CAD build for the part. Positions are in the model's coordinates, mm. Round coordinates to 2 decimals unless told otherwise and drop trailing zeros. Answer as CSV lines item,"result". Start each with the question number.
from build123d import *

# Parameters (mm, degrees)
SKETCH_R  = 2.1
PAD_DEPTH = 800


with BuildPart() as part:
    # Sketch → Pad (new body)
    with BuildSketch(Plane.XY):
        with BuildLine():
            Line((-10, 4.58), (-10, 9.5))
            ThreePointArc((-9.5, 10), (-9.853553, 9.853553), (-10, 9.5))
            Line((-9.5, 10), (-4.58, 10))
            Line((-4.58, 10), (-3.125, 8.545))
            Line((-3.125, 8.545), (-3.125, 8.2))
            Line((-5.5, 8.2), (-3.125, 8.2))
            Line((-5.5, 8.2), (-5.5, 6.56066))
            Line((-5.5, 6.56066), (-2.83934, 3.9))
            Line((-0.125, 3.9), (-2.83934, 3.9))
            ThreePointArc((-0.125, 3.9), (0, 3.775), (0.125, 3.9))
            Line((0.125, 3.9), (2.83934, 3.9))
            Line((2.83934, 3.9), (5.5, 6.56066))
            Line((5.5, 6.56066), (5.5, 8.2))
            Line((5.5, 8.2), (3.125, 8.2))
            Line((3.125, 8.2), (3.125, 8.545))
            Line((3.125, 8.545), (4.58, 10))
            Line((4.58, 10), (15.42, 10))
            Line((15.42, 10), (16.875, 8.545))
            Line((16.875, 8.545), (16.875, 8.2))
            Line((16.875, 8.2), (14.5, 8.2))
            Line((14.5, 8.2), (14.5, 6.56066))
            Line((14.5, 6.56066), (17.16066, 3.9))
            Line((17.16066, 3.9), (19.875, 3.9))
            ThreePointArc((19.875, 3.9), (20, 3.775), (20.125, 3.9))
            Line((20.125, 3.9), (22.83934, 3.9))
            Line((22.83934, 3.9), (25.5, 6.56066))
            Line((25.5, 6.56066), (25.5, 8.2))
            Line((25.5, 8.2), (23.125, 8.2))
            Line((23.125, 8.2), (23.125, 8.545))
            Line((23.125, 8.545), (24.58, 10))
            Line((24.58, 10), (29.5, 10))
            ThreePointArc((30, 9.5), (29.853554, 9.853554), (29.5, 10))
            Line((30, 9.5), (30, 4.58))
            Line((30, 4.58), (28.545, 3.125))
            Line((28.545, 3.125), (28.2, 3.125))
            Line((28.2, 3.125), (28.2, 5.5))
            Line((28.2, 5.5), (26.560661, 5.5))
            Line((26.560661, 5.5), (23.9, 2.83934))
            Line((23.9, 2.83934), (23.9, 0.125))
            ThreePointArc((23.9, 0.125), (23.775, 2e-06), (23.899997, -0.125))
            Line((23.899997, -2.83934), (23.899997, -0.125))
            Line((26.560658, -5.5), (23.899997, -2.83934))
            Line((28.199997, -5.5), (26.560658, -5.5))
            Line((28.199997, -3.125), (28.199997, -5.5))
            Line((28.544997, -3.125), (28.199997, -3.125))
            Line((29.999997, -4.58), (28.544997, -3.125))
            Line((29.999997, -9.5), (29.999997, -4.58))
            ThreePointArc((29.5, -10), (29.853552, -9.853552), (29.999997, -9.5))
            Line((24.58, -10), (29.5, -10))
            Line((23.125, -8.545), (24.58, -10))
            Line((23.125, -8.2), (23.125, -8.545))
            Line((25.5, -8.2), (23.125, -8.2))
            Line((25.5, -6.56066), (25.5, -8.2))
            Line((22.83934, -3.9), (25.5, -6.56066))
            Line((20.125, -3.9), (22.83934, -3.9))
            ThreePointArc((20.125, -3.9), (20, -3.775), (19.875, -3.9))
            Line((17.16066, -3.9), (19.875, -3.9))
            Line((14.5, -6.56066), (17.16066, -3.9))
            Line((14.5, -8.2), (14.5, -6.56066))
            Line((16.875, -8.2), (14.5, -8.2))
            Line((16.875, -8.545), (16.875, -8.2))
            Line((15.42, -10), (16.875, -8.545))
            Line((4.58, -10), (15.42, -10))
            Line((4.58, -10), (3.125, -8.545))
            Line((3.125, -8.545), (3.125, -8.2))
            Line((3.125, -8.2), (5.5, -8.2))
            Line((5.5, -8.2), (5.5, -6.56066))
            Line((2.83934, -3.9), (5.5, -6.56066))
            Line((0.125, -3.9), (2.83934, -3.9))
            ThreePointArc((0.125, -3.9), (0, -3.775), (-0.125, -3.9))
            Line((-0.125, -3.9), (-2.83934, -3.9))
            Line((-2.83934, -3.9), (-5.5, -6.56066))
            Line((-5.5, -6.56066), (-5.5, -8.2))
            Line((-5.5, -8.2), (-3.125, -8.2))
            Line((-3.125, -8.545), (-3.125, -8.2))
            Line((-4.58, -10), (-3.125, -8.545))
            Line((-9.5, -10), (-4.58, -10))
            ThreePointArc((-10, -9.5), (-9.853553, -9.853553), (-9.5, -10))
            Line((-10, -4.58), (-10, -9.5))
            Line((-8.545, -3.125), (-10, -4.58))
            Line((-8.2, -3.125), (-8.545, -3.125))
            Line((-8.2, -5.5), (-8.2, -3.125))
            Line((-6.56066, -5.5), (-8.2, -5.5))
            Line((-3.9, -2.83934), (-6.56066, -5.5))
            Line((-3.9, -0.125), (-3.9, -2.83934))
            ThreePointArc((-3.9, -0.125), (-3.775, 0), (-3.9, 0.125))
            Line((-3.9, 2.83934), (-3.9, 0.125))
            Line((-6.56066, 5.5), (-3.9, 2.83934))
            Line((-8.2, 5.5), (-6.56066, 5.5))
            Line((-8.2, 5.5), (-8.2, 3.125))
            Line((-8.545, 3.125), (-8.2, 3.125))
            Line((-10, 4.58), (-8.545, 3.125))
        make_face()
        Circle(SKETCH_R, mode=Mode.SUBTRACT)
        with Locations((20, 0)):
            Circle(SKETCH_R, mode=Mode.SUBTRACT)
        with BuildLine():
            Line((7, 5.93934), (3.9, 2.83934))
            Line((3.9, 2.83934), (3.9, 0.125))
            ThreePointArc((3.9, 0.125), (3.775, 0), (3.9, -0.125))
            Line((3.9, -0.125), (3.9, -2.83934))
            Line((3.9, -2.83934), (7, -5.93934))
            Line((7, -5.93934), (7, -8.2))
            Line((7, -8.2), (13, -8.2))
            Line((13, -8.2), (13, -5.93934))
            Line((13, -5.93934), (16.1, -2.83934))
            Line((16.1, -2.83934), (16.1, -0.125))
            ThreePointArc((16.1, -0.125), (16.224999, 0), (16.1, 0.125))
            Line((16.1, 2.83934), (16.1, 0.125))
            Line((13, 5.93934), (16.1, 2.83934))
            Line((13, 8.2), (13, 5.93934))
            Line((7, 8.2), (13, 8.2))
            Line((7, 5.93934), (7, 8.2))
        make_face(mode=Mode.SUBTRACT)
    extrude(amount=PAD_DEPTH)


solid = part.part
Item 1: Probe line 1 (X direction, y = 6.75, z = 449.5); line 2 (X direction, y = -1, z = 495.5); line 3 (Y direction, x = 20, z = 322) (3 decimals). List the from-to ranges inside material, lowest first.
Item 2: Pin check, flat tips, straight feed: pin 1 (1.4 mm diameter, centred on x = 19, z = 546.5, fed in from -Y); pin 2 (2 mm diameter, centred on y = -1.5, z = 233.5, fed in from +X); pin 3 (3 mm diameter, centred on x = -2.5, z = 127.5, fed in from +Y). Stop position of each tip, or through.
Item 3: Band-saw the part on A-A, the plane z = 278.5. Count the separate pieces of the cut face and the enclosed holes in it, and give its area (3 significant figures).
Values:
1,line 1,"-10 to -5.5, 5.5 to 7, 13 to 14.5, 25.5 to 30"
1,line 2,"-3.9 to -1.85, 1.85 to 3.9, 16.1 to 18.15, 21.85 to 23.9"
1,line 3,"-3.775 to -2.1, 2.1 to 3.775"
2,pin 1,"y = -3.9"
2,pin 2,"x = 23.9"
2,pin 3,"y = 9.42"
3,separate pieces,"1"
3,enclosed holes,"3"
3,area,"298 mm²"
